Can you work these out from the model? Positions are in its coordinate system, mm. Round coordinates to 2 decimals unless told otherwise and drop trailing zeros. Loops run counter-clockwise (first coordinate to the right, second up) from the corner with the lowest first, then second, coordinate; pieces in that order, holes last. Notation, with made-up numbers: M 72.25,78 L 79.25,78 A20 ccw 79.25,113 Z; hole C -33.5,65 d5. An arc over 180 degrees is marked long. Return JSON: item names as keys, results as strings.
```python
from build123d import *

# Parameters (mm, degrees)
SKETCH1_W           = 69
SKETCH1_H           = 35
BOSS_EXTRUDE1_DEPTH = 3
FILLET4_R           = 2
CUT_EXTRUDE1_REACH  = 40.801
SKETCH2_R           = 1.8


with BuildPart() as part:
    # Sketch1 → Boss-Extrude1 (new body)
    with BuildSketch(Plane(origin=(0, 0, 0), x_dir=(1, 0, 0), z_dir=(0, 1, 0))):
        Rectangle(SKETCH1_W, SKETCH1_H)
    extrude(amount=BOSS_EXTRUDE1_DEPTH)

    # Fillet4
    fillet4_edges = [part.edges().sort_by_distance(p)[0] for p in [
        (-34.5, 1.5, 17.5),
        (-34.5, 1.5, -17.5),
    ]]
    fillet(fillet4_edges, radius=FILLET4_R)

    # Sketch2 → Cut-Extrude1 (cut, up to next)
    with BuildSketch(Plane.XZ, mode=Mode.PRIVATE) as cut_extrude1_sk1:
        with Locations(Location((-29, 14.625, 0), (0, 0, 270))):
            Circle(SKETCH2_R)
    cut_extrude1_tool1 = extrude(cut_extrude1_sk1.sketch, amount=-CUT_EXTRUDE1_REACH, mode=Mode.PRIVATE) & part.part
    # Sketch2 → Cut-Extrude1 (cut, up to next)
    with BuildSketch(Plane.XZ, mode=Mode.PRIVATE) as cut_extrude1_sk2:
        with Locations(Location((29, -14.898327821, 0), (0, 0, 270))):
            Circle(SKETCH2_R)
    cut_extrude1_tool2 = extrude(cut_extrude1_sk2.sketch, amount=-CUT_EXTRUDE1_REACH, mode=Mode.PRIVATE) & part.part
    add(cut_extrude1_tool1.solids().sort_by_distance((-29, 0, 14.625))[0], mode=Mode.SUBTRACT)
    add(cut_extrude1_tool2.solids().sort_by_distance((29, 0, -14.898328))[0], mode=Mode.SUBTRACT)


solid = part.part
```
Q1. If I drill on line 1 along X through (y, z) = (1.25, 14); line 2 along Z through (x, y) = (-28, 1.8); line 3 along X through (y, z) = (1.95, 15), over which ranges is the centre line in solid material (lowest first)?
Results:
{"line 1": "x = -34.5 to -30.69, -27.31 to 34.5", "line 2": "z = -17.5 to 13.13, 16.12 to 17.5", "line 3": "x = -34.5 to -30.76, -27.24 to 34.5"}
Q2. Thinking about a two-plate mould opening in Z: for faces 1 (the cylindrical face through (-33.93, 1.52, 16.9)), 2 (the cylindrical face through (30.785, 1.479, -14.664)), 3 (the flat face through (34.5, 1, 0)), which applies, pulls with the +Z half, pulls with the -Z half, needs draft (parallel to the pull), parting line crosses it, or undercut?
Results:
{"face 1": "pulls with the +Z half", "face 2": "undercut", "face 3": "needs draft"}
Q3. Suppose I cut it at A-A, the plane x = -29. Please give me the cut outline in (y, z) (3 decimals), plus the area to 3 significant figures.
Results:
{"outline": "M 0,-17.5 L 3,-17.5 L 3,12.825 L 0,12.825 Z; M 0,16.425 L 3,16.425 L 3,17.5 L 0,17.5 Z", "area": "94.2 mm2"}
